Could you check a few things on this model? Use its own coordinates, in mm. Face numbers are marked on the shaded views. Give positions to 0.01 mm unless a question says otherwise; leave off trailing zeros. Order: outer loops, then holes, each group sorted by start corner. A loop starts at its lowest first (then second) coordinate and runs counter-clockwise, first axis right, second up. Notation, with made-up numbers: M 7.25,29.25 L 39.25,29.25 A27 cw 39.25,66.25 Z; hole C -13,-16 d6. An arc over 180 degrees is marked long. Use a Markdown table: item, result. Add a question column.
Item 1: Suppose I cut it at C-C on y = 58. Write out the boundary of the cut face in (x, z).
Item 2: Suppose I cut it at A-A on x = 0. Write out the boundary of the cut face in (y, z).
Item 3: I'm going to push flat-ended pins straight in: pin 1 Ø17.5 at (x, z) = (-3, 12) entering from +Y; pin 2 Ø1.5 at (x, z) = (-32, 20) entering from +Y; pin 3 Ø4.5 at (x, y) = (-3, 76.5) entering from +Z. Where does each tip first touch, or does it pass through?
Item 4: If we mould it in two halves opening along X, with no side actions, what happens to the marked faces 1, 2 and 3? For each: released by +X, released by -X, zero draft, split by the parting line, or undercut.
Item 5: If I drill on L1, parallel to Y at x = 0, z = 35.6; L2, parallel to Z at x = 0, y = 44; L3, parallel to Y at x = 7.5, z = 8, over which ranges is the centre line in solid material (lowest first)? Write a range as from..to.
Item 6: Suppose I cut it at B-B on z = 0. Write out the boundary of the cut face in (x, y).
from build123d import *
from build123d.topology import SkipClean

# Parameters (mm, degrees)
SKETCH1_R           = 40
BOSS_EXTRUDE1_DEPTH = 5
SKETCH2_R           = 40
SKETCH2_R_2         = 34
BOSS_EXTRUDE2_DEPTH = 60
BOSS_EXTRUDE3_DEPTH = 20
FILLET1_R           = 5
SKETCH4_R           = 3
CUT_EXTRUDE1_DEPTH  = 95
FILLET2_R           = 5
FILLET3_R           = 5


with BuildPart() as part:
    # Sketch1 → Boss-Extrude1 (new body)
    with BuildSketch(Plane(origin=(0, 0, 0), x_dir=(1, 0, 0), z_dir=(0, 1, 0))):
        with Locations(Location((0, 0, 0), (0, 0, 270))):
            Circle(SKETCH1_R)
    extrude(amount=BOSS_EXTRUDE1_DEPTH)

    # Sketch2 → Boss-Extrude2 (add)
    with BuildSketch(Plane(origin=(0, 5, 0), x_dir=(1, 0, 0), z_dir=(0, 1, 0))):
        with Locations(Location((0, 0, 0), (0, 0, 270))):
            Circle(SKETCH2_R)
        with Locations(Location((0, 0, 0), (0, 0, 270))):
            Circle(SKETCH2_R_2, mode=Mode.SUBTRACT)
    extrude(amount=BOSS_EXTRUDE2_DEPTH)

    # Sketch3 → Boss-Extrude3 (add)
    with SkipClean():  # the faces are left unmerged after this step: merging them gives an invalid solid
        with BuildSketch(Plane(origin=(0, 65, 0), x_dir=(1, 0, 0), z_dir=(0, 1, 0))):
            with BuildLine():
                ThreePointArc((8.738415, -32.857877), (0, -34), (-8.738415, -32.857877))
                Line((-8.738415, -32.857877), (-8.738415, -39.027584))
                Line((-8.738415, -39.027584), (8.738415, -39.027584))
                Line((8.738415, -39.027584), (8.738415, -32.857877))
            make_face()
            with BuildLine():
                Line((8.738415, 39.027584), (-8.738415, 39.027584))
                Line((-8.738415, 39.027584), (-8.738415, 32.857877))
                ThreePointArc((-8.738415, 32.857877), (0, 34), (8.738415, 32.857877))
                Line((8.738415, 32.857877), (8.738415, 39.027584))
            make_face()
        extrude(amount=BOSS_EXTRUDE3_DEPTH)

    # Fillet1
    # the kernel refuses this fillet: 5 mm, written as the material it adds along each edge
    with BuildSketch(Plane(origin=(8.738415, 65, 39.027584), x_dir=(1, 0, 0), z_dir=(0, 0, -1))) as fillet1_piece_1_section:
        with BuildLine():
            CenterArc((FILLET1_R, -FILLET1_R), FILLET1_R, 90, 90)
            Line((0, -FILLET1_R), (0, 0))
            Line((0, 0), (FILLET1_R, 0))
        make_face()
    fillet1_piece_1 = extrude(amount=18.669707, mode=Mode.PRIVATE)
    fillet1_piece_1 = fillet1_piece_1 & Plane(origin=(0, 66.126044, 0), x_dir=(0, 0, 1), z_dir=(0, -1, 0)) * Cylinder(40, 58, mode=Mode.PRIVATE)
    fillet1_piece_1 = fillet1_piece_1 - Plane(origin=(0, 66.126044, 0), x_dir=(0, 0, 1), z_dir=(0, -1, 0)) * Cylinder(34, 58, mode=Mode.PRIVATE)
    add(fillet1_piece_1)
    with BuildSketch(Plane(origin=(-8.738415, 65, 20.357877), x_dir=(-1, 0, 0), z_dir=(0, 0, 1))) as fillet1_piece_2_section:
        with BuildLine():
            CenterArc((FILLET1_R, -FILLET1_R), FILLET1_R, 90, 90)
            Line((0, -FILLET1_R), (0, 0))
            Line((0, 0), (FILLET1_R, 0))
        make_face()
    fillet1_piece_2 = extrude(amount=18.669707, mode=Mode.PRIVATE)
    fillet1_piece_2 = fillet1_piece_2 & Plane(origin=(0, 66.126045, 0), x_dir=(0, 0, 1), z_dir=(0, -1, 0)) * Cylinder(40, 58, mode=Mode.PRIVATE)
    fillet1_piece_2 = fillet1_piece_2 - Plane(origin=(0, 66.126045, 0), x_dir=(0, 0, 1), z_dir=(0, -1, 0)) * Cylinder(34, 58, mode=Mode.PRIVATE)
    add(fillet1_piece_2)
    with BuildSketch(Plane(origin=(-8.738415, 65, -39.027584), x_dir=(-1, 0, 0), z_dir=(0, 0, 1))) as fillet1_piece_3_section:
        with BuildLine():
            CenterArc((FILLET1_R, -FILLET1_R), FILLET1_R, 90, 90)
            Line((0, -FILLET1_R), (0, 0))
            Line((0, 0), (FILLET1_R, 0))
        make_face()
    fillet1_piece_3 = extrude(amount=18.669707, mode=Mode.PRIVATE)
    fillet1_piece_3 = fillet1_piece_3 & Plane(origin=(0, 66.126044, 0), x_dir=(0, 0, 1), z_dir=(0, -1, 0)) * Cylinder(40, 58, mode=Mode.PRIVATE)
    fillet1_piece_3 = fillet1_piece_3 - Plane(origin=(0, 66.126044, 0), x_dir=(0, 0, 1), z_dir=(0, -1, 0)) * Cylinder(34, 58, mode=Mode.PRIVATE)
    add(fillet1_piece_3)
    with BuildSketch(Plane(origin=(8.738415, 65, -20.357877), x_dir=(1, 0, 0), z_dir=(0, 0, -1))) as fillet1_piece_4_section:
        with BuildLine():
            CenterArc((FILLET1_R, -FILLET1_R), FILLET1_R, 90, 90)
            Line((0, -FILLET1_R), (0, 0))
            Line((0, 0), (FILLET1_R, 0))
        make_face()
    fillet1_piece_4 = extrude(amount=18.669707, mode=Mode.PRIVATE)
    fillet1_piece_4 = fillet1_piece_4 & Plane(origin=(0, 66.126045, 0), x_dir=(0, 0, 1), z_dir=(0, -1, 0)) * Cylinder(40, 58, mode=Mode.PRIVATE)
    fillet1_piece_4 = fillet1_piece_4 - Plane(origin=(0, 66.126045, 0), x_dir=(0, 0, 1), z_dir=(0, -1, 0)) * Cylinder(34, 58, mode=Mode.PRIVATE)
    add(fillet1_piece_4)

    # Sketch4 → Cut-Extrude1 (cut)
    with BuildSketch(Plane(origin=(0, 0, -39.027584), x_dir=(-1, 0, 0), z_dir=(0, 0, -1))):
        with Locations((0, 77.048027)):
            Circle(SKETCH4_R)
    extrude(amount=-CUT_EXTRUDE1_DEPTH, mode=Mode.SUBTRACT)

    # Fillet2
    fillet2_edges = [part.edges().sort_by_distance(p)[0] for p in [
        (0, 5, -34),
    ]]
    fillet(fillet2_edges, radius=FILLET2_R)

    # Fillet3
    # the kernel refuses this fillet: 5 mm, written as the material it adds along each edge
    with BuildSketch(Plane(origin=(-8.738415, 65, 39.027584), x_dir=(0, 1, 0), z_dir=(1, 0, 0))) as fillet3_piece_1_section:
        with BuildLine():
            CenterArc((FILLET3_R, FILLET3_R), FILLET3_R, 180, 90)
            Line((0, FILLET3_R), (0, 0))
            Line((0, 0), (FILLET3_R, 0))
        make_face()
    fillet3_piece_1 = extrude(amount=30.004694, mode=Mode.PRIVATE)
    fillet3_piece_1 = fillet3_piece_1 & Plane(origin=(0, 66.676029, 0), x_dir=(0, 0, 1), z_dir=(0, -1, 0)) * Cylinder(40, 81, mode=Mode.PRIVATE)
    fillet3_piece_1 = fillet3_piece_1 - Plane(origin=(13.738415, 70, 39.364377), x_dir=(1, 0, 0), z_dir=(0, 0, 1)) * Cylinder(5, 81, mode=Mode.PRIVATE)
    add(fillet3_piece_1)
    with BuildSketch(Plane(origin=(8.738415, 65, -39.027584), x_dir=(0, 1, 0), z_dir=(-1, 0, 0))) as fillet3_piece_2_section:
        with BuildLine():
            CenterArc((FILLET3_R, FILLET3_R), FILLET3_R, 180, 90)
            Line((0, FILLET3_R), (0, 0))
            Line((0, 0), (FILLET3_R, 0))
        make_face()
    fillet3_piece_2 = extrude(amount=30.004694, mode=Mode.PRIVATE)
    fillet3_piece_2 = fillet3_piece_2 - Plane(origin=(-13.738415, 70, -39.364375), x_dir=(-1, 0, 0), z_dir=(0, 0, -1)) * Cylinder(5, 81, mode=Mode.PRIVATE)
    fillet3_piece_2 = fillet3_piece_2 & Plane(origin=(0, 66.676016, 0), x_dir=(0, 0, 1), z_dir=(0, -1, 0)) * Cylinder(40, 81, mode=Mode.PRIVATE)
    add(fillet3_piece_2)
    with BuildSketch(Plane(origin=(8.738415, 65, -39.027584), x_dir=(0, 0, -1), z_dir=(1, 0, 0))) as fillet3_piece_3_section:
        with BuildLine():
            CenterArc((FILLET3_R, FILLET3_R), FILLET3_R, 180, 90)
            Line((0, FILLET3_R), (0, 0))
            Line((0, 0), (FILLET3_R, 0))
        make_face()
    fillet3_piece_3 = extrude(amount=12.527864, mode=Mode.PRIVATE)
    fillet3_piece_3 = fillet3_piece_3 & Plane(origin=(0, 67.353955, 0), x_dir=(0, 0, 1), z_dir=(0, -1, 0)) * Cylinder(40, 46, mode=Mode.PRIVATE)
    fillet3_piece_3 = fillet3_piece_3 - Plane(origin=(13.738415, 70, -39.02968), x_dir=(1, 0, 0), z_dir=(0, 0, 1)) * Cylinder(5, 46, mode=Mode.PRIVATE)
    add(fillet3_piece_3)
    with BuildSketch(Plane(origin=(-8.738415, 65, 39.027584), x_dir=(0, 1, 0), z_dir=(-1, 0, 0))) as fillet3_piece_4_section:
        with BuildLine():
            CenterArc((FILLET3_R, -FILLET3_R), FILLET3_R, 90, 90)
            Line((0, -FILLET3_R), (0, 0))
            Line((0, 0), (FILLET3_R, 0))
        make_face()
    fillet3_piece_4 = extrude(amount=12.527864, mode=Mode.PRIVATE)
    fillet3_piece_4 = fillet3_piece_4 - Plane(origin=(-13.738415, 70, 39.02968), x_dir=(-1, 0, 0), z_dir=(0, 0, -1)) * Cylinder(5, 46, mode=Mode.PRIVATE)
    fillet3_piece_4 = fillet3_piece_4 & Plane(origin=(0, 67.353955, 0), x_dir=(0, 0, 1), z_dir=(0, -1, 0)) * Cylinder(40, 46, mode=Mode.PRIVATE)
    add(fillet3_piece_4)


solid = part.part
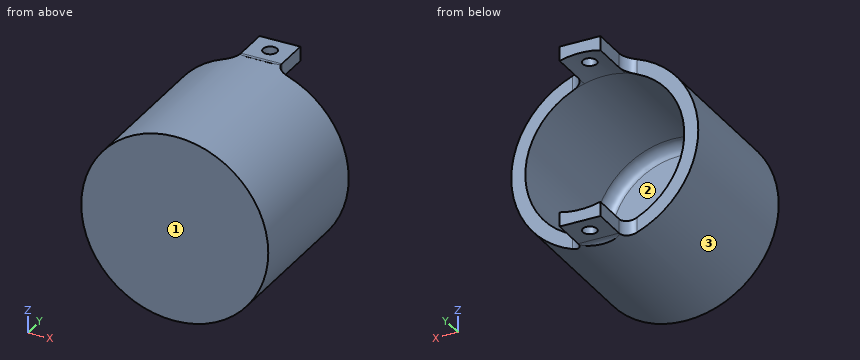
Findings below:
| question | item | result |
|---|---|---|
| 1 | outline | C 0,0 d80; hole C 0,0 d68 |
| 2 | outline | M 0,-40 L 67.04,-40 A5 cw 70,-39.03 L 74.05,-39.03 L 74.05,-34 L 10,-34 A5 cw 5,-29 L 5,29 A5 cw 10,34 L 74.05,34 L 74.05,39.03 L 70,39.03 A5 cw 67.04,40 L 0,40 Z; M 80.05,-39.03 L 85,-39.03 L 85,-34 L 80.05,-34 Z; M 80.05,34 L 85,34 L 85,39.03 L 80.05,39.03 Z |
| 3 | pin 1 | stops at y = 5 |
| 3 | pin 2 | stops at y = 65 |
| 3 | pin 3 | stops at z = 39.03 |
| 4 | face 1 | zero draft |
| 4 | face 2 | undercut |
| 4 | face 3 | split by the parting line |
| 5 | L1 | y = 0..74.05, 80.05..85 |
| 5 | L2 | z = -40..-34, 34..40 |
| 5 | L3 | y = 0..5 |
| 6 | outline | M -40,0 L 40,0 L 40,65 L 34,65 L 34,10 A5 cw 29,5 L -29,5 A5 cw -34,10 L -34,65 L -40,65 Z |
